from build123d import *

# Parameters (mm, degrees)
F2_DEPTH = 5.9
F3_SIZE  = 1


with BuildPart() as f2:
    # F1 (on Top) → F2 (new body)
    with BuildSketch(Plane.XY):
        Polygon((4.6730719134, -54.0581345186), (11.6730719134, -54.0581345186), (11.6730719134, -59.9581345186), (24.6730719134, -59.9581345186), (24.6730719134, -54.0581345186), (24.6730719134, 25.9418654814), (24.6730719134, 31.8418654814), (11.6730719134, 31.8418654814), (11.6730719134, 25.9418654814), (4.6730719134, 25.9418654814), (4.6730719134, -11.1581345186), (11.6730719134, -11.1581345186), (11.6730719134, -16.9581345186), (4.6730719134, -16.9581345186), align=None)
    extrude(amount=F2_DEPTH)

    # F3
    f3_edges = [f2.edges().sort_by_distance(p)[0] for p in [
        (4.673072, -11.158135, 2.95),
        (4.673072, -16.958135, 2.95),
    ]]
    chamfer(f3_edges, length=F3_SIZE)


solid = f2.part
The listing builds one solid part. Answer for the finished solid, in the listing's coordinates (mm). A direction names the side the tool comes from. Give positions to 0.01 mm unless a question says otherwise; leave off trailing zeros. Loops run counter-clockwise (first coordinate to the right, second up) from the corner with the lowest first, then second, coordinate; pieces in that order, holes last. Notation, with made-up numbers: (59.25, 59) - (81.25, 59) arc R12 ccw to (81.25, 64) - close; hole circle Ø2 at (56.5, 22). An arc over 180 degrees is marked (long way). Use one line per item in the form item = value.
1. Section A-A on z = 0.8 is taken. Give the vertices of the cut face in (x, y), then the cut area to 3 significant figures.
Calculated:
outline = (4.67, -54.06) - (11.67, -54.06) - (11.67, -59.96) - (24.67, -59.96) - (24.67, 31.84) - (11.67, 31.84) - (11.67, 25.94) - (4.67, 25.94) - (4.67, -10.16) - (5.67, -11.16) - (11.67, -11.16) - (11.67, -16.96) - (5.67, -16.96) - (4.67, -17.96) - close
area = 1,710 mm^2
2. Find the intervals of material crossed by line 1 along Y through (x, z) = (10, 4.9), in increasing order. Write a range as [from, to].
Calculated:
line_1 = [-54.06, -16.96], [-11.16, 25.94]
3. Which of the six approach directions +Z, -Z, +X, -X, +Y, -Y give full straight-line access (tool end or side, diameter ignored) to faces 1 (the face through (15, -13, 5.9)), 2 (the face through (11.673, -14, 3)), 3 (the face through (11.673, -57, 3)), 4 (the face through (8, 25.942, 3))?
Calculated:
face_1 = +Z, +X, -X, +Y, -Y
face_2 = +Z, -Z, -X
face_3 = +Z, -Z, -X, -Y
face_4 = +Z, -Z, -X, +Y
4. The mould has two halves that part along Y. Classify faces 5 (the face through (8, -54.058, 3)), 6 (the face through (4.673, -36, 3)), 7 (the face through (9, -11.158, 3)): pulls with the +Y half, pulls with the -Y half, needs draft (parallel to the pull), parting line crosses it, or undercut.
Calculated:
face_5 = pulls with the -Y half
face_6 = needs draft
face_7 = undercut
5. Section B-B on y = -12 is taken. Give the vertices of the cut face in (x, z), then the cut area to 3 significant figures.
Calculated:
outline = (11.67, 0) - (24.67, 0) - (24.67, 5.9) - (11.67, 5.9) - close
area = 76.7 mm^2
6. Given pin 1 Ø1.8 at (x, z) = (10, 2) entering from -Y; pin 2 Ø3 at (x, z) = (10, 2.5) entering from +Y, each flat-ended and moving along its own axis, determine where each tip first touches the part or whether it passes through.
Calculated:
pin_1 = -54.06
pin_2 = 25.94
